Here's the drawing with two shaded views (mm, measured from the low corner). I have some questions. A direction names the side the tool comes from. Give positions to 0.01 mm unless a question says otherwise; leave off trailing zeros. Loops run counter-clockwise (first coordinate to the right, second up) from the corner with the lowest first, then second, coordinate; pieces in that order, holes last. Notation, with made-up numbers: M -24.75,24.5 L 2.25,24.5 A29 ccw 2.25,58.5 Z; hole C 63.5,11 d9. An arc over 180 degrees is marked long. Answer in a Markdown table with one row per item. Add a question column.
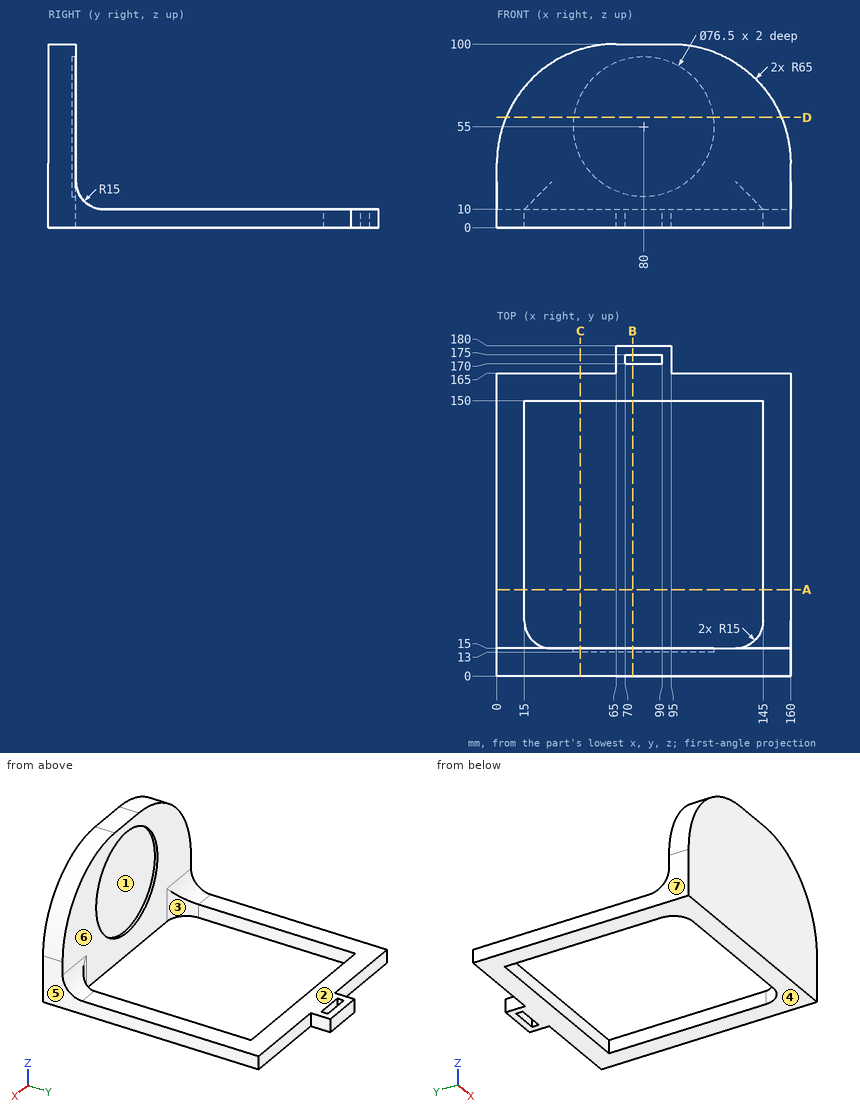
Item 1: Suppose I cut it at D-D (z = 60). List the corners of the cut face in (x, y) for me, then the cut area to 3 significant figures.
Item 2: Suppose I cut it at A-A (y = 47). List the corners of the cut face in (x, z) for me, then the cut area to 3 significant figures.
Item 3: For P1, Ø10, axis at x = 63, z = 22.5, coming from the -Y side; P2, Ø1, axis at x = 107, z = 51, coming from the +Y side; P3, Ø5.5, axis at y = 172, z = 5, coming from the -X side; P4, Ø8, axis at x = 115, z = 2.5, coming from the +Y side, each with a flat end and sliding along its axis, tell me the tip position at first contact or that it passes through.
Item 4: If we mould it in two halves opening along X, with no side actions, what happens to the marked faces 4, 5, 6 and 7? For each: +X half, -X half, draft (parallel to the pull), parting line (faces both ways), or undercut.
Item 5: Suppose I cut it at C-C (x = 45.5). List the corners of the cut face in (y, z) for me.
Item 6: Suppose I cut it at B-B (x = 74). List the corners of the cut face in (y, z) for me, then the cut area to 3 significant figures.
Item 7: I need wall thicknesses on L1, parallel to Z at x = 80, y = 14.45; L2, parallel to Y at x = 120, z = 19.5; L3, parallel to Y at x = 61.5, z = 27.5. Which ranges of each line are inside material? Lowest first, please.
Item 8: For the marked faces 1, 2 and 3, which set-ups out of +Z, -Z, +X, -X, +Y, -Y let a thin tool reach every point of the face, with its end or its side?
Values found:
| question | item | result |
|---|---|---|
| 1 | outline | M 5,0 L 155,0 L 155,15 L 117.92,15 L 117.92,13 L 42.08,13 L 42.08,15 L 5,15 Z |
| 1 | area | 2,100 mm² |
| 2 | outline | M 0,0 L 15,0 L 15,10 L 0,10 Z; M 145,0 L 160,0 L 160,10 L 145,10 Z |
| 2 | area | 300 mm² |
| 3 | P1 | y = 0 |
| 3 | P2 | y = 13 |
| 3 | P3 | x = 65 |
| 3 | P4 | y = 165 |
| 4 | face 4 | draft |
| 4 | face 5 | +X half |
| 4 | face 6 | undercut |
| 4 | face 7 | -X half |
| 5 | outline | M 0,0 L 15,0 L 15,38.48 L 13,38.48 L 13,71.52 L 15,71.52 L 15,97.01 L 0,97.01 Z; M 150,0 L 165,0 L 165,10 L 150,10 Z |
| 6 | outline | M 0,0 L 15,0 L 15,17.22 L 13,17.22 L 13,92.78 L 15,92.78 L 15,100 L 0,100 Z; M 150,0 L 170,0 L 170,10 L 150,10 Z; M 175,0 L 180,0 L 180,10 L 175,10 Z |
| 6 | area | 1,600 mm² |
| 7 | L1 | 0 to 16.75, 93.25 to 100 |
| 7 | L2 | 0 to 15 |
| 7 | L3 | 0 to 13 |
| 8 | face 1 | +Y |
| 8 | face 2 | +Z, +X, -X, +Y |
| 8 | face 3 | +Z, -Z |
